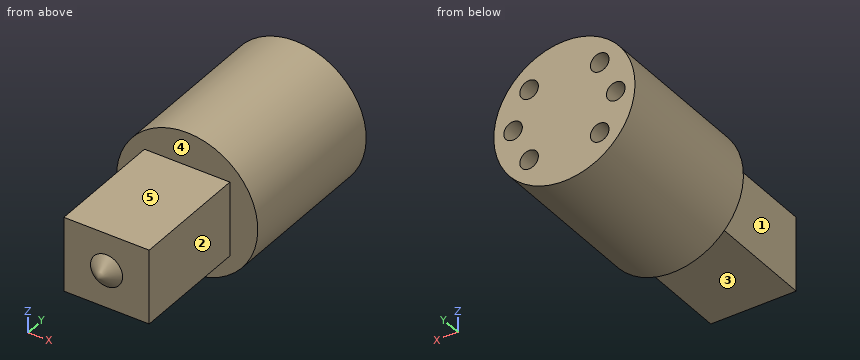
from build123d import *

# Parameters (mm, degrees)
SKETCH2_R                  = 11
BOSS_EXTRUDE1_DEPTH        = 25
SKETCH3_W                  = 13.3
SKETCH3_H                  = 11.6
BOSS_EXTRUDE2_DEPTH        = 18.6
M2_5_CLEARANCE_HOLE1_D     = 2.9
M2_5_CLEARANCE_HOLE1_DEPTH = 5
M2_5_CLEARANCE_HOLE1_TIP   = 0.871247898


with BuildPart() as part:
    # Sketch2 → Boss-Extrude1 (new body)
    with BuildSketch(Plane(origin=(0, 0, 0), x_dir=(1, 0, 0), z_dir=(0, 1, 0))):
        with Locations(Location((0, 0, 0), (0, 0, 270))):
            Circle(SKETCH2_R)
    extrude(amount=-BOSS_EXTRUDE1_DEPTH)

    # Sketch3 → Boss-Extrude2 (add)
    with BuildSketch(Plane.XZ.offset(25)):
        Rectangle(SKETCH3_W, SKETCH3_H)
    extrude(amount=BOSS_EXTRUDE2_DEPTH)

    # Sketch4 → Revolve1 (revolve)
    with BuildSketch(Plane.XY):
        Polygon((-2.5, -43.6), (0, -45.6), (0, -43.6), align=None)
    revolve(axis=Axis((0, -45.6, 0), (0, 1, 0)))

    # M2.5 Clearance Hole1
    with Locations(Plane(origin=(0, 0, 0), x_dir=(1, 0, 0), z_dir=(0, 1, 0))):
        with Locations((-5.5, 5.5), (5.5, -5.5), (-5.5, -5.5), (5.5, 5.5), (8, 0), (-8, 0)):
            Hole(M2_5_CLEARANCE_HOLE1_D / 2, depth=M2_5_CLEARANCE_HOLE1_DEPTH)
            with Locations((0, 0, -(M2_5_CLEARANCE_HOLE1_DEPTH + M2_5_CLEARANCE_HOLE1_TIP / 2))):  # 118° drill point
                Cone(0, M2_5_CLEARANCE_HOLE1_D / 2, M2_5_CLEARANCE_HOLE1_TIP, mode=Mode.SUBTRACT)


solid = part.part
Read the model definition and answer for the solid it produces. Units are mm, in the model's axes. Face numbers are marked on the shaded views. A direction names the side the tool comes from. Give positions to 0.01 mm unless a question says otherwise; leave off trailing zeros. Loops run counter-clockwise (first coordinate to the right, second up) from the corner with the lowest first, then second, coordinate; pieces in that order, holes last. Notation, with made-up numbers: M -37.75,-2.75 L -16.75,-2.75 A20 ccw -16.75,9.25 Z; hole C 16.25,79 d4. An arc over 180 degrees is marked long. Write each question's results on one line, items separated by ' | '.
1. A tool of negligible diameter and unlimited length cuts with its end or side. For the marked faces 1, 2, 3, 4 and 5, from which of +Z, -Z, +X, -X, +Y, -Y can it reach the whole face along a straight path? Write none if from no direction.
Values:
face 1: +Z, -Z, -X, -Y | face 2: +Z, -Z, +X, -Y | face 3: -Z, +X, -X, -Y | face 4: -Y | face 5: +Z, +X, -X, -Y
2. Given pin 1 (4 mm diameter, centred on x = 8, z = 0, fed in from -Y); pin 2 (1 mm diameter, centred on x = 8, z = 0.5, fed in from +Y); pin 3 (3 mm diameter, centred on x = -8.5, y = -30, fed in from +Z) (1 decimal); pin 4 (2.5 mm diameter, centred on x = -8, z = 0, fed in from +Y), each flat-ended and moving along its own axis, determine where each tip first touches the part or whether it passes through.
Values:
pin 1: stops at y = -43.6 | pin 2: stops at y = -5.27 | pin 3: passes through | pin 4: stops at y = -5.12
3. Section B-B on y = -23 is taken. Give the vertices of the cut face in (x, z), plus the area to 3 significant figures.
Values:
outline: C 0,0 d22 | area: 380 mm^2
4. Section C-C on z = 3 is taken. Give the vertices of the cut face in (x, y).
Values:
outline: M -10.58,-25 L -6.65,-25 L -6.65,-43.6 L 6.65,-43.6 L 6.65,-25 L 10.58,-25 L 10.58,0 L -10.58,0 Z
5. Section D-D on y = -32 is taken. Give the vertices of the cut face in (x, z).
Values:
outline: M -6.65,-5.8 L 6.65,-5.8 L 6.65,5.8 L -6.65,5.8 Z
6. Straight lines are drawn through the part: line 1 (Z direction, x = 5.5, y = -4); line 2 (X direction, y = -32.5, z = 0.5). For each, find the intervals that lie inside material, in ascending order. Write a range as [from, to].
Values:
line 1: z = [-9.53, -6.95], [-4.05, 4.05], [6.95, 9.53] | line 2: x = [-6.65, 6.65]
7. Section A-A on x = -3.5 is taken. Give the vertices of the cut face in (y, z).
Values:
outline: M -43.6,-5.8 L -25,-5.8 L -25,-10.43 L 0,-10.43 L 0,10.43 L -25,10.43 L -25,5.8 L -43.6,5.8 Z
